Source: three-view drawing plus pictorial views. Frame: mm from the lowest corner of the part. A direction names the side the tool comes from. Give positions to 0.01 mm unless a question says otherwise; leave off trailing zeros. Order: outer loops, then holes, each group sorted by start corner. A loop starts at its lowest first (then second) coordinate and runs counter-clockwise, first axis right, second up. Notation, with made-up numbers: M 54,-22 L 87,-22 A24 cw 87,3 Z; hole C -5,3.5 d2. An arc over 180 degrees is marked long. One line per item, written item: value. Start each with the question number.
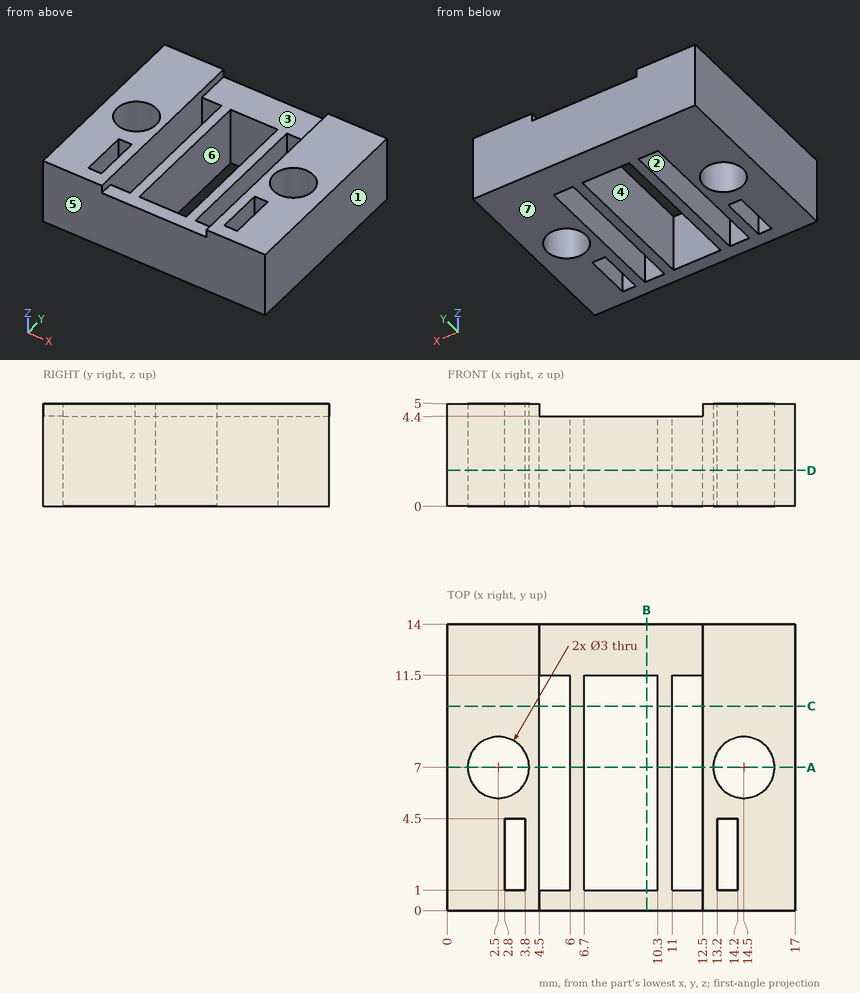
Q1. Ray query, line 1 along X through (y, z) = (2, 3.45); line 2 along Y through (x, z) = (12.25, 0.55); line 3 along Y through (x, z) = (2.5, 1.05). Return the intervals inside material, ascending. Write a range as [from, to].
Q2. Section query B-B on x = 9.75. Return loops of the section in (y, z).
Q3. Mould query, pull axis Y, two halves, no side actions, for the marked faces 4, 5, 6 and 7. Classes: +Y half, -Y half, draft (parallel to the pull), parting line (faces both ways), or undercut.
Q4. Section query D-D on z = 1.75. Return loops of the section in (x, y).
Q5. Set-up query: the marked faces 1, 2 and 3. Return all of +Z, -Z, +X, -X, +Y, -Y with unobstructed straight access to the full face (end or side cutting, diameter ignored); none if empty.
Q6. Section query C-C on y = 10. Return loops of the section in (x, z), and give its area (3 significant figures).
Q7. Section query A-A on y = 7. Return loops of the section in (x, z), and give its area (3 significant figures).
Results below:
1. line 1: [0, 2.8], [3.8, 4.5], [6, 6.7], [10.3, 11], [12.5, 13.2], [14.2, 17]
1. line 2: [0, 1], [11.5, 14]
1. line 3: [0, 5.5], [8.5, 14]
2. outline: M 0,0 L 1,0 L 1,4.4 L 0,4.4 Z; M 11.5,0 L 14,0 L 14,4.4 L 11.5,4.4 Z
3. face 4: undercut
3. face 5: -Y half
3. face 6: undercut
3. face 7: draft
4. outline: M 0,0 L 17,0 L 17,14 L 0,14 Z; hole C 2.5,7 d3; hole M 2.8,1 L 3.8,1 L 3.8,4.5 L 2.8,4.5 Z; hole M 4.5,1 L 6,1 L 6,11.5 L 4.5,11.5 Z; hole M 6.7,1 L 10.3,1 L 10.3,11.5 L 6.7,11.5 Z; hole M 11,1 L 12.5,1 L 12.5,11.5 L 11,11.5 Z; hole C 14.5,7 d3; hole M 13.2,1 L 14.2,1 L 14.2,4.5 L 13.2,4.5 Z
5. face 1: +Z, -Z, +X, +Y, -Y
5. face 2: +Z, -Z
5. face 3: +Z, +Y, -Y
6. outline: M 0,0 L 4.5,0 L 4.5,5 L 0,5 Z; M 6,0 L 6.7,0 L 6.7,4.4 L 6,4.4 Z; M 10.3,0 L 11,0 L 11,4.4 L 10.3,4.4 Z; M 12.5,0 L 17,0 L 17,5 L 12.5,5 Z
6. area: 51.2 mm2
7. outline: M 0,0 L 1,0 L 1,5 L 0,5 Z; M 4,0 L 4.5,0 L 4.5,5 L 4,5 Z; M 6,0 L 6.7,0 L 6.7,4.4 L 6,4.4 Z; M 10.3,0 L 11,0 L 11,4.4 L 10.3,4.4 Z; M 12.5,0 L 13,0 L 13,5 L 12.5,5 Z; M 16,0 L 17,0 L 17,5 L 16,5 Z
7. area: 21.2 mm2
